Geometry: final body of the model. Coordinates: model frame, mm. A direction names the side the tool comes from. Coordinates: 2 decimals unless noted, no trailing zeros. Write each loop counter-clockwise with the first axis right and the second up, starting at its lowest first coordinate (ties: lowest second). Pieces come first, ordered by that corner, then holes.
from build123d import *

# Parameters (mm, degrees)
SKETCH2_OUTSIDE_W   = 37.554
SKETCH2_OUTSIDE_H   = 37.554
CUT_EXTRUDE1_DEPTH  = 74.1
SKETCH3_OUTSIDE_W   = 37.554
SKETCH3_OUTSIDE_H   = 37.554
SKETCH3_OUTSIDE_W_2 = 1
SKETCH3_OUTSIDE_H_2 = 17.972200756
CUT_EXTRUDE2_DEPTH  = 0.2
SKETCH4_OUTSIDE_W   = 37.554
SKETCH4_OUTSIDE_H   = 37.554
CUT_EXTRUDE3_DEPTH  = 3
SKETCH5_OUTSIDE_W   = 37.554
SKETCH5_OUTSIDE_H   = 37.554
CUT_EXTRUDE4_DEPTH  = 3.5


with BuildPart() as part:
    # Sketch1 → Revolve1 (revolve)
    with BuildSketch(Plane.XY):
        with BuildLine():
            Line((0, 0), (0, 9))
            Line((0, 9), (1.2, 9))
            Line((1.2, 9), (1.2, 5.25))
            ThreePointArc((1.2, 5.25), (1.492893219, 4.542893219), (2.2, 4.25))
            Line((2.2, 4.25), (7.2, 4.25))
            ThreePointArc((7.2, 4.25), (7.970049199, 4.299619825), (8.72736183, 4.44765859))
            Line((8.72736183, 4.44765859), (17.67263817, 6.80234141))
            ThreePointArc((17.67263817, 6.80234141), (18.429950801, 6.950380175), (19.2, 7))
            Line((19.2, 7), (52.5, 7))
            Line((52.5, 7), (56, 4))
            Line((56, 4), (59.5, 7))
            Line((59.5, 7), (75.3, 7))
            Line((75.3, 7), (75.3, 7.5))
            Line((75.3, 7.5), (76.5, 7.5))
            Line((76.5, 7.5), (76.5, 4))
            Line((76.5, 4), (79.5, 4))
            Line((79.5, 4), (79.5, 5))
            Line((79.5, 5), (81.3, 5))
            Line((81.3, 5), (84, 0))
            Line((84, 0), (0, 0))
        make_face()
    revolve(axis=Axis((84, 0, 0), (-1, 0, 0)))

    # Sketch2 outside → Cut-Extrude1 (cut)
    with BuildSketch(Plane(origin=(1.2, 0, 0), x_dir=(0, 0, -1), z_dir=(1, 0, 0))):
        Rectangle(SKETCH2_OUTSIDE_W, SKETCH2_OUTSIDE_H)
        with BuildLine():
            Line((-0.6, 8.979977728), (-0.6, 0.6))
            Line((-0.6, 0.6), (-8.979977728, 0.6))
            ThreePointArc((-8.979977728, 0.6), (-9, 0), (-8.979977728, -0.6))
            Line((-8.979977728, -0.6), (-0.6, -0.6))
            Line((-0.6, -0.6), (-0.6, -8.979977728))
            ThreePointArc((-0.6, -8.979977728), (0, -9), (0.6, -8.979977728))
            Line((0.6, -8.979977728), (0.6, -0.6))
            Line((0.6, -0.6), (8.979977728, -0.6))
            ThreePointArc((8.979977728, -0.6), (9, 0), (8.979977728, 0.6))
            Line((8.979977728, 0.6), (0.6, 0.6))
            Line((0.6, 0.6), (0.6, 8.979977728))
            ThreePointArc((0.6, 8.979977728), (0, 9), (-0.6, 8.979977728))
        make_face(mode=Mode.SUBTRACT)
    extrude(amount=CUT_EXTRUDE1_DEPTH, mode=Mode.SUBTRACT)

    # Sketch3 outside → Cut-Extrude2 (cut)
    with BuildSketch(Plane.ZY):
        Rectangle(SKETCH3_OUTSIDE_W, SKETCH3_OUTSIDE_H)
        with Locations((2.25, 0)):
            Rectangle(SKETCH3_OUTSIDE_W_2, SKETCH3_OUTSIDE_H_2, mode=Mode.SUBTRACT)
        Rectangle(SKETCH3_OUTSIDE_W_2, SKETCH3_OUTSIDE_H_2, mode=Mode.SUBTRACT)
        with Locations((4.5, 0)):
            Rectangle(SKETCH3_OUTSIDE_W_2, SKETCH3_OUTSIDE_H_2, mode=Mode.SUBTRACT)
        with Locations((6.75, 0)):
            Rectangle(SKETCH3_OUTSIDE_W_2, SKETCH3_OUTSIDE_H_2, mode=Mode.SUBTRACT)
        with Locations((9, 0)):
            Rectangle(SKETCH3_OUTSIDE_W_2, SKETCH3_OUTSIDE_H_2, mode=Mode.SUBTRACT)
        with Locations((11.25, 0)):
            Rectangle(SKETCH3_OUTSIDE_W_2, SKETCH3_OUTSIDE_H_2, mode=Mode.SUBTRACT)
        with Locations((13.5, 0)):
            Rectangle(SKETCH3_OUTSIDE_W_2, SKETCH3_OUTSIDE_H_2, mode=Mode.SUBTRACT)
        with Locations((-2.25, 0)):
            Rectangle(SKETCH3_OUTSIDE_W_2, SKETCH3_OUTSIDE_H_2, mode=Mode.SUBTRACT)
        with Locations((-4.5, 0)):
            Rectangle(SKETCH3_OUTSIDE_W_2, SKETCH3_OUTSIDE_H_2, mode=Mode.SUBTRACT)
        with Locations((-6.75, 0)):
            Rectangle(SKETCH3_OUTSIDE_W_2, SKETCH3_OUTSIDE_H_2, mode=Mode.SUBTRACT)
        with Locations((-9, 0)):
            Rectangle(SKETCH3_OUTSIDE_W_2, SKETCH3_OUTSIDE_H_2, mode=Mode.SUBTRACT)
        with Locations((-11.25, 0)):
            Rectangle(SKETCH3_OUTSIDE_W_2, SKETCH3_OUTSIDE_H_2, mode=Mode.SUBTRACT)
        with Locations((-13.5, 0)):
            Rectangle(SKETCH3_OUTSIDE_W_2, SKETCH3_OUTSIDE_H_2, mode=Mode.SUBTRACT)
    extrude(amount=-CUT_EXTRUDE2_DEPTH, mode=Mode.SUBTRACT)

    # Sketch4 outside → Cut-Extrude3 (cut)
    with BuildSketch(Plane(origin=(76.5, 0, 0), x_dir=(0, 0, -1), z_dir=(1, 0, 0))):
        Rectangle(SKETCH4_OUTSIDE_W, SKETCH4_OUTSIDE_H)
        with BuildLine():
            Line((0.6, 0.6), (0.6, 8.979977728))
            ThreePointArc((0.6, 8.979977728), (0, 9), (-0.6, 8.979977728))
            Line((-0.6, 8.979977728), (-0.6, 0.6))
            Line((-0.6, 0.6), (-8.979977728, 0.6))
            ThreePointArc((-8.979977728, 0.6), (-9, 0), (-8.979977728, -0.6))
            Line((-8.979977728, -0.6), (-0.6, -0.6))
            Line((-0.6, -0.6), (-0.6, -8.979977728))
            ThreePointArc((-0.6, -8.979977728), (0, -9), (0.6, -8.979977728))
            Line((0.6, -8.979977728), (0.6, -0.6))
            Line((0.6, -0.6), (8.979977728, -0.6))
            ThreePointArc((8.979977728, -0.6), (9, 0), (8.979977728, 0.6))
            Line((8.979977728, 0.6), (0.6, 0.6))
        make_face(mode=Mode.SUBTRACT)
    extrude(amount=CUT_EXTRUDE3_DEPTH, mode=Mode.SUBTRACT)

    # Sketch5 outside → Cut-Extrude4 (cut)
    with BuildSketch(Plane(origin=(84, 0, 0), x_dir=(0, 0, -1), z_dir=(1, 0, 0))):
        Rectangle(SKETCH5_OUTSIDE_W, SKETCH5_OUTSIDE_H)
        with BuildLine():
            Line((0.6, 0.6), (0.6, 4.711952886))
            ThreePointArc((0.6, 4.711952886), (0, 4.75), (-0.6, 4.711952886))
            Line((-0.6, 4.711952886), (-0.6, 0.6))
            Line((-0.6, 0.6), (-4.711952886, 0.6))
            ThreePointArc((-4.711952886, 0.6), (-4.75, 0), (-4.711952886, -0.6))
            Line((-4.711952886, -0.6), (-0.6, -0.6))
            Line((-0.6, -0.6), (-0.6, -4.711952886))
            ThreePointArc((-0.6, -4.711952886), (0, -4.75), (0.6, -4.711952886))
            Line((0.6, -4.711952886), (0.6, -0.6))
            Line((0.6, -0.6), (4.711952886, -0.6))
            ThreePointArc((4.711952886, -0.6), (4.75, 0), (4.711952886, 0.6))
            Line((4.711952886, 0.6), (0.6, 0.6))
        make_face(mode=Mode.SUBTRACT)
    extrude(amount=-CUT_EXTRUDE4_DEPTH, mode=Mode.SUBTRACT)


solid = part.part
Item 1: Section B-B, the plane x = 6. Output: boundary loops of the cut face in (y, z).
Derived:
outline: (-4.21, -0.6) - (-0.6, -0.6) - (-0.6, -4.21) arc R4.25 ccw to (0.6, -4.21) - (0.6, -0.6) - (4.21, -0.6) arc R4.25 ccw to (4.21, 0.6) - (0.6, 0.6) - (0.6, 4.21) arc R4.25 ccw to (-0.6, 4.21) - (-0.6, 0.6) - (-4.21, 0.6) arc R4.25 ccw to start
Item 2: Set-up query: faces 1 (the flat face through (38, -0.6, 4)), 2 (the flat face through (78, 2, 0.6)), 3 (the conical face through (13.26, -5.64, -0.01)), 4 (the cylindrical face through (80.01, -1.08, 4.88)). Return all of +Z, -Z, +X, -X, +Y, -Y with unobstructed straight access to the full face (end or side cutting, diameter ignored); none if empty.
Derived:
face 1: +Z, -Y
face 2: +Z, +Y
face 3: -Y
face 4: +X
Item 3: Pin query (flat end, axial travel): pin 1 (4 mm diameter, centred on x = 41.5, z = -5, fed in from +Y); pin 2 (2.5 mm diameter, centred on x = 81.5, z = -3, fed in from -Y); pin 3 (5 mm diameter, centred on x = 53, y = -4.5, fed in from +Z). Return the tip coordinate at first contact, or that it passes through.
Derived:
pin 1: stops at y = 0.6
pin 2: stops at y = -4.47
pin 3: stops at z = 0.6
Item 4: Pull-direction query (X, two-part tool) for faces 5 (the flat face through (82, 2, 0.6)), 6 (the conical face through (57.774, 0.012, -5.521)), 7 (the flat face through (76.5, 2, 2)); classes: released by +X, released by -X, zero draft, split by the parting line, or undercut.
Derived:
face 5: zero draft
face 6: undercut
face 7: undercut
Item 5: Section A-A, the plane x = 37.5. Output: boundary loops of the cut face in (y, z), plus the area to 3 significant figures.
Derived:
outline: (-6.97, -0.6) - (-0.6, -0.6) - (-0.6, -6.97) arc R7 ccw to (0.6, -6.97) - (0.6, -0.6) - (6.97, -0.6) arc R7 ccw to (6.97, 0.6) - (0.6, 0.6) - (0.6, 6.97) arc R7 ccw to (-0.6, 6.97) - (-0.6, 0.6) - (-6.97, 0.6) arc R7 ccw to start
area: 32.1 mm2
Item 6: Material intervals for probe 1 along X at (y, z) = (-1, -3); probe 2 along X at (y, z) = (7.25, -1.25); probe 3 along Y at (x, z) = (47, 5.5), sorted ascending.
Derived:
probe 1: x = 0.2 to 1.2, 75.3 to 76.5, 79.5 to 80.5
probe 2: x = 0.2 to 1.2, 75.3 to 76.5
probe 3: y = -0.6 to 0.6
